Source: CAD feature listing. Evaluate the final solid. Frame: model axes, mm. Face numbers are marked on the shaded views. A direction names the side the tool comes from. Round coordinates to 2 decimals unless told otherwise and drop trailing zeros. Order: outer loops, then holes, each group sorted by start corner. A loop starts at its lowest first (then second) coordinate and runs counter-clockwise, first axis right, second up. Notation, with made-up numbers: M 61,-32 L 76,-32 A27 cw 76,-11 Z; hole C 60,59 d4. An arc over 180 degrees is marked long. Answer as CSV lines item,"result". Start each with the question number.
Item 1: Set-up query: the marked faces 1 and 2. Return all of +Z, -Z, +X, -X, +Y, -Y with unobstructed straight access to the full face (end or side cutting, diameter ignored); none if empty.
Item 2: Section query D-D on z = 1050.5. Return the cut outline in (x, y), plus the area to 3 significant figures.
Item 3: Section query A-A on x = 282. Return the cut outline in (y, z).
Item 4: Line query: line 1 (X direction, y = -147.5, z = 813.5); line 2 (X direction, y = -297, z = 883); line 3 (Z direction, x = 706, y = -184.5). Output: solid intervals per line, ascending. Write a range as [from, to].
Item 5: Section query B-B on z = -199.5. Return the cut outline in (x, y), plus the area to 3 significant figures.
Item 6: Pull-direction query (Z, two-part tool) for the marked faces 3, 4 and 5; classes: +Z half, -Z half, draft (parallel to the pull), parting line (faces both ways), or undercut.
Item 7: Section query C-C on y = -32. Return the cut outline in (x, z).
Item 8: First-contact query: P1, Ø12, axis at x = 328.5, z = 343.5, coming from the +Y side; P2, Ø12, axis at y = -143, z = 656, coming from the -X side; P3, Ø8, axis at x = 54.5, y = -150, coming from the +Z side; P4, Ø10, axis at y = -242.5, z = -310, coming from the +X side. Flat tips, straight axial feed; report the tip coordinate or a pass-through.
from build123d import *

# Parameters (mm, degrees)
F1_DEPTH = 400


with BuildPart() as f1:
    # F0 (on Front) → F1 (new body)
    with BuildSketch(Plane.XZ):
        Polygon((-99.569657, -448.701831), (-272.774738, -548.701831), (1727.225262, -548.701831), (1554.020181, -448.701831), align=None)
        Polygon((727.225262, 1183.348976), (-272.774738, -548.701831), (-99.569657, -448.701831), (727.225262, 983.348976), align=None)
        Polygon((1554.020181, -448.701831), (1727.225262, -548.701831), (727.225262, 1183.348976), (727.225262, 983.348976), align=None)
    extrude(amount=F1_DEPTH)


solid = f1.part
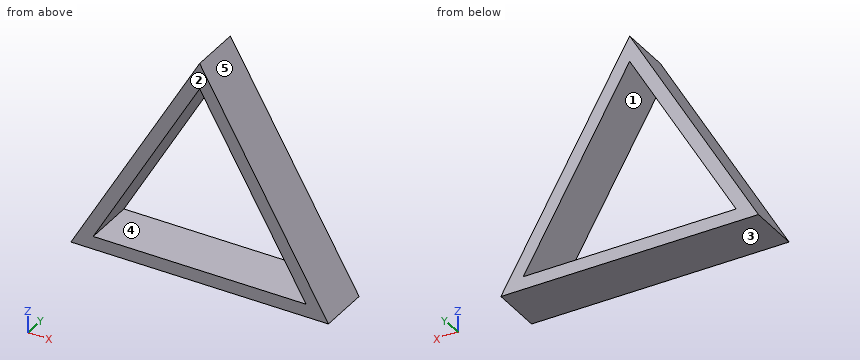
Results:
1,face 1,"+Y, -Y"
1,face 2,"+Z, -Z, +X, -X, -Y"
2,outline,"M 650.52,-400 L 803.93,-400 L 803.93,0 L 650.52,0 Z"
2,area,"61,400 mm^2"
3,outline,"M -400,-548.7 L 0,-548.7 L 0,-448.7 L -400,-448.7 Z; M -400,212.2 L 0,212.2 L 0,412.2 L -400,412.2 Z"
4,line 1,"[513.69, 629.16], [825.29, 940.76]"
4,line 2,"[553.82, 669.29], [785.16, 900.63]"
4,line 3,"[-548.7, -448.7], [946.59, 1146.59]"
5,outline,"M -71.16,-400 L 44.31,-400 L 44.31,0 L -71.16,0 Z; M 1410.14,-400 L 1525.61,-400 L 1525.61,0 L 1410.14,0 Z"
5,area,"92,400 mm^2"
6,face 3,"-Z half"
6,face 4,"undercut"
6,face 5,"+Z half"
7,outline,"M -272.77,-548.7 L 1727.23,-548.7 L 727.23,1183.35 Z; hole M -99.57,-448.7 L 1554.02,-448.7 L 727.23,983.35 Z"
8,P1,"y = 0"
8,P2,"x = 419.3"
8,P3,"z = 25.08"
8,P4,"x = 1592.3"
